Build history of the part. All positions in model axes, mm. A direction names the side the tool comes from. Give positions to 0.01 mm unless a question says otherwise; leave off trailing zeros. Loops run counter-clockwise (first coordinate to the right, second up) from the corner with the lowest first, then second, coordinate; pieces in that order, holes last. Notation, with made-up numbers: (44, 40) -> (98, 40) arc R26 ccw to (98, 64) -> close; hole circle Ø9 at (9.5, -2.5). An arc over 180 degrees is marked (long way). One line per question, with ' | ' between items. Start each with the question number.
(1) Slice it at D-D, the plane z = -40. Write the cut outline in (x, y), then the cut area to 3 significant figures.
(2) Slice it at B-B, the plane z = 0. Write the cut outline in (x, y), then the cut area to 3 significant figures.
(3) Mould opens along Y. For faces 1 (the face through (1, 3, -20)), 2 (the face through (1, -2, 0)), 3 (the face through (-2, 0, -19)) say: pulls with the +Y half, pulls with the -Y half, needs draft (parallel to the pull), parting line crosses it, or undercut.
(4) Drill centre lines: L1, parallel to Y at x = -4.2, z = 0; L2, parallel to X at y = -2.75, z = -32; L3, parallel to Y at x = -1, z = -20.5. Where is each one in solid material? Low to high. Write a range as from..to.
(5) Slice it at A-A, the plane x = -2.5. Write the cut outline in (y, z).
(6) Flat gauge pins, fed straight in: pin 1 Ø3 at (x, z) = (-4.5, -7.5) entering from -Y; pin 2 Ø8 at (x, z) = (1.5, -33.5) entering from -Y; pin 3 Ø3 at (y, z) = (-2.5, -0.5) entering from -X. Where does each tip first touch, or does it go through?
(7) 3-axis set-ups, long thin cutter, end or side, ignore diameter. For faces 4 (the face through (-4.27, 3.2, -4.22)), 5 (the face through (-4.27, -3.29, -35.04)), 6 (the face through (-1.5, -0.4, -21)): which of +Z, -Z, +X, -X, +Y, -Y reach the whole face in a straight line?
```python
from build123d import *
from build123d.topology import SkipClean

# Parameters (mm, degrees)
SKETCH_1_R                  = 5
SKETCH_1_W                  = 40
SKETCH_1_H                  = 6
EXTRUDE_1_DEPTH             = 2.5
CUT_EXTRUDE_2_DEPTH         = 46.467021015
CUT_EXTRUDE_2_DEPTH_BACK    = 46.467021015
SKETCH_1_3_R                = 2
FILLET_1_R                  = 3
EXTRUDE_START               = -1.5
EXTRUDE_2_DEPTH             = 1.5
SKETCH_2_R                  = 1.8
EXTRUDE_4_DEPTH             = 5
EXTRUDE_5_REACH             = 48.014
SKETCH_1_5_R                = 2
EXTRUDE_5_DIRECTION_2_REACH = 48.014
SKETCH_3_W                  = 2
SKETCH_3_H                  = 3
EXTRUDE_8_DEPTH             = 1.5
SKETCH_4_W                  = 0.5
SKETCH_4_H                  = 1.5
EXTRUDE_9_DEPTH             = 2


with BuildPart() as part:
    # Sketch 1 → Extrude 1 (new body)
    with BuildSketch(Plane(origin=(0, 0, 0), x_dir=(0, 0, -1), z_dir=(1, 0, 0))):
        Circle(SKETCH_1_R)
        with Locations((40, -1)):
            Circle(SKETCH_1_R)
        with Locations((20, 0)):
            Rectangle(SKETCH_1_W, SKETCH_1_H)
    extrude(amount=EXTRUDE_1_DEPTH)

    # Sketch 1_3 → Cut-Extrude 2 (cut, two sides: drawn at the far end of the back side and taken through both)
    with BuildSketch(Plane(origin=(0, 0, 0), x_dir=(0, 0, -1), z_dir=(1, 0, 0)).offset(-CUT_EXTRUDE_2_DEPTH_BACK)):
        Circle(SKETCH_1_3_R)
        with Locations((40, -1)):
            Circle(SKETCH_1_3_R)
    extrude(amount=CUT_EXTRUDE_2_DEPTH + CUT_EXTRUDE_2_DEPTH_BACK, mode=Mode.SUBTRACT)

    # Fillet 1
    fillet_1_edges = [part.edges().sort_by_distance(p)[0] for p in [
        (1.25, -3, -35.417424305),
        (1.25, 3, -37),
        (1.25, 3, -4),
        (1.25, -3, -4),
    ]]
    fillet(fillet_1_edges, radius=FILLET_1_R)

    # Sketch 1_4 → Extrude 2 (add)
    with SkipClean():  # the faces are left unmerged after this step: merging them gives an invalid solid
        with BuildSketch(Plane(origin=(0, 0, 0), x_dir=(0, 0, -1), z_dir=(1, 0, 0)).offset(EXTRUDE_START)):
            with BuildLine():
                ThreePointArc((37, 3), (35.16534763, 0.275200556), (35.417424305, -3))
                Line((35.417424305, -3), (40, -3))
                ThreePointArc((40, -3), (38, -1), (40, 1))
                Line((40, 1), (40, 3))
                Line((40, 3), (37, 3))
            make_face()
            with BuildLine():
                Line((40, -3), (35.417424305, -3))
                ThreePointArc((35.417424305, -3), (41.021548218, -5.894531565), (45, -1))
                ThreePointArc((45, -1), (42.236067977, 3.472135955), (37, 3))
                Line((37, 3), (40, 3))
                Line((40, 3), (40, 1))
                ThreePointArc((40, 1), (41.414213562, 0.414213562), (42, -1))
                ThreePointArc((42, -1), (41.414213562, -2.414213562), (40, -3))
            make_face()
        extrude(amount=EXTRUDE_2_DEPTH)

    # Extrude 5: up to this face of the body (flat: up to its plane)
    extrude_5_end = Plane(part.part.faces().sort_by_distance((2.5, -0.197791912, -20.041492076))[0])
    # Sketch 1_5 → Extrude 5 (add, up to the picked face)
    with BuildSketch(Plane(origin=(0, 0, 0), x_dir=(0, 0, -1), z_dir=(1, 0, 0)), mode=Mode.PRIVATE) as extrude_5_sk1:
        with Locations((40, -1)):
            Circle(SKETCH_1_5_R)
    extrude_5_tool1 = split(extrude(extrude_5_sk1.sketch, amount=EXTRUDE_5_REACH, mode=Mode.PRIVATE), bisect_by=extrude_5_end, keep=Keep.BOTH, mode=Mode.PRIVATE)


with BuildPart() as body_2:
    # Sketch 2 → Extrude 4 (new body)
    with BuildSketch(Plane(origin=(2.5, 0, 0), x_dir=(0, 0, -1), z_dir=(1, 0, 0))):
        with Locations((40, -1)):
            Circle(SKETCH_2_R)
    extrude(amount=EXTRUDE_4_DEPTH)


with BuildPart() as part_1:
    add(part.part)

    add(body_2.part)  # Extrude 5 merges body 2
    add(extrude_5_tool1.solids().sort_by(Axis((0, -1, -40), (1, 0, 0)))[0])

    # Extrude 5 direction 2: up to this face of the body (flat: up to its plane)
    extrude_5_direction_2_end = Plane(part_1.part.faces().sort_by_distance((-1.5, -3.141421356, -40))[0])
    # Sketch 1_5 → Extrude 5 direction 2 (add, up to the picked face)
    with BuildSketch(Plane(origin=(0, 0, 0), x_dir=(0, 0, -1), z_dir=(1, 0, 0)), mode=Mode.PRIVATE) as extrude_5_direction_2_sk1:
        with Locations((40, -1)):
            Circle(SKETCH_1_5_R)
    extrude_5_direction_2_tool1 = split(extrude(extrude_5_direction_2_sk1.sketch, amount=-EXTRUDE_5_DIRECTION_2_REACH, mode=Mode.PRIVATE), bisect_by=extrude_5_direction_2_end, keep=Keep.BOTH, mode=Mode.PRIVATE)
    add(extrude_5_direction_2_tool1.solids().sort_by(Axis((0, -1, -40), (-1, 0, 0)))[0])

    # Sketch 3 → Extrude 8 (add)
    with BuildSketch(Plane.ZY):
        with Locations((-20, 0)):
            Rectangle(SKETCH_3_W, SKETCH_3_H)
    extrude(amount=EXTRUDE_8_DEPTH)

    # Sketch 4 → Extrude 9 (add)
    with BuildSketch(Plane(origin=(0, 0, -21), x_dir=(-1, 0, 0), z_dir=(0, 0, -1))):
        with Locations((1.25, 0.75)):
            Rectangle(SKETCH_4_W, SKETCH_4_H)
    extrude(amount=EXTRUDE_9_DEPTH)

    # Mirror 3: part across plane


with BuildPart() as part_2:
    add(part_1.part)
    add(part_1.part.mirror(Plane.ZY.offset(1.5)))


solid = part_2.part
```
Final values:
1) outline: (-10.5, -2.8) -> (-5.5, -2.8) -> (-5.5, -6) -> (2.5, -6) -> (2.5, -2.8) -> (7.5, -2.8) -> (7.5, 0.8) -> (2.5, 0.8) -> (2.5, 4) -> (-5.5, 4) -> (-5.5, 0.8) -> (-10.5, 0.8) -> close | area: 116 mm2
2) outline: (-5.5, -5) -> (-3, -5) -> (-3, -2) -> (-5.5, -2) -> close; (-5.5, 2) -> (-3, 2) -> (-3, 5) -> (-5.5, 5) -> close; (0, -5) -> (2.5, -5) -> (2.5, -2) -> (0, -2) -> close; (0, 2) -> (2.5, 2) -> (2.5, 5) -> (0, 5) -> close | area: 30.0 mm2
3) face 1: pulls with the +Y half | face 2: undercut | face 3: needs draft
4) L1: -5..-2, 2..5 | L2: -5.5..-3, 0..2.5 | L3: -1.5..1.5
5) outline: circle Ø10 at (-1, -40); (-1.5, -21) -> (1.5, -21) -> (1.5, -19) -> (-1.5, -19) -> close
6) pin 1: y = -3 | pin 2: y = -5.33 | pin 3: x = -5.5
7) face 4: +X, -X, +Y | face 5: +X, -X, -Y | face 6: -Y
